Input: dimensioned drawing with shaded views. Units: mm. Origin: part minimum x, y, z. Give positions to 0.01 mm unless a question says otherwise; leave off trailing zeros. Write each loop counter-clockwise with the first axis right and the second up, starting at its lowest first coordinate (ties: lowest second). Pieces come first, ordered by that corner, then holes.
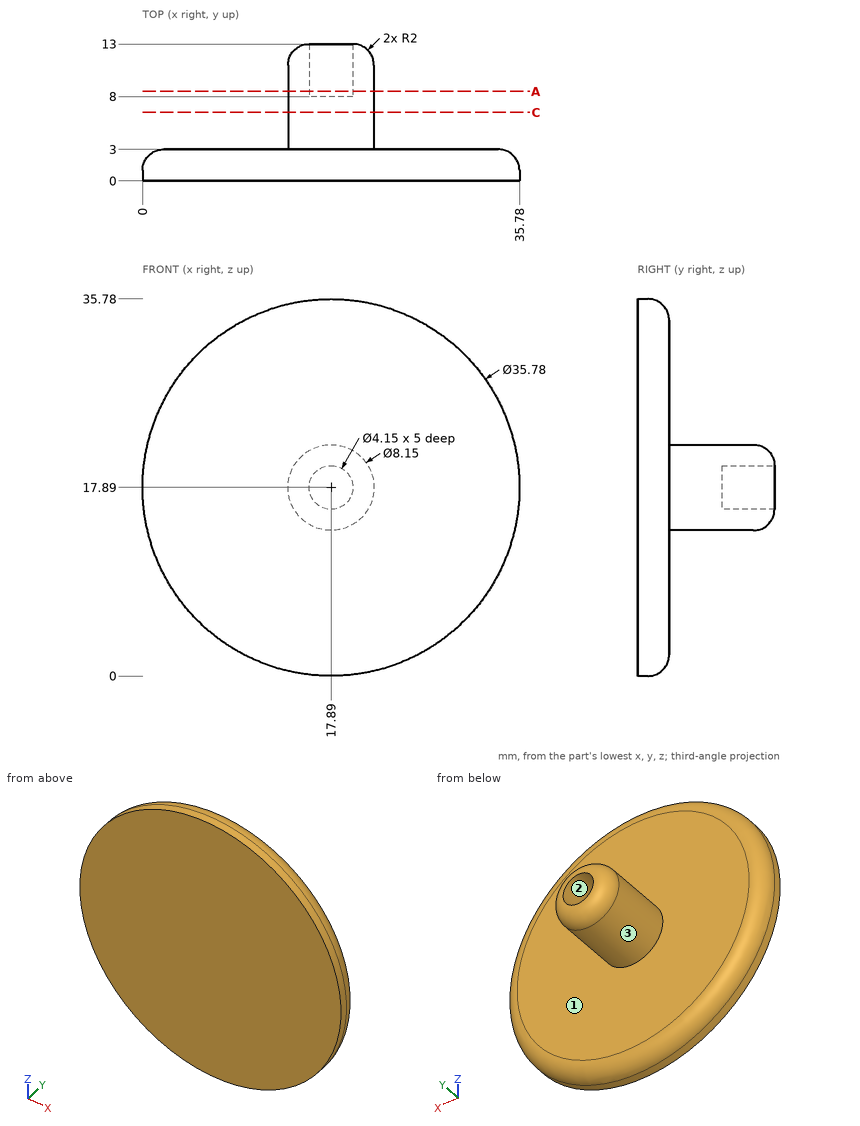
Item 1: Pin query (flat end, axial travel): pin 1 Ø5 at (x, y) = (5.5, 7.5) entering from -Z; pin 2 Ø1.5 at (x, z) = (25.5, 3.5) entering from +Y. Return the tip coordinate at first contact, or that it passes through.
Found:
pin 1: passes through
pin 2: stops at y = 3
Item 2: Section C-C, the plane y = 6.5. Return the cut outline in (x, z) (3 decimals).
Found:
outline: circle Ø8.15 at (17.89, 17.89)
Item 3: Line query: L1, parallel to X at y = 10.9, z = 17.89 (3 decimals); L2, parallel to Z at x = 18, y = 10; L3, parallel to Z at x = 18, y = 3.5. Output: solid intervals per line, ascending.
Found:
L1: x = 13.815 to 15.815, 19.965 to 21.965
L2: z = 13.82 to 15.82, 19.96 to 21.96
L3: z = 13.82 to 21.96
Item 4: Section A-A, the plane y = 8.5. Return the cut outline in (x, z) (3 decimals).
Found:
outline: circle Ø8.15 at (17.89, 17.89); hole circle Ø4.15 at (17.89, 17.89)
Item 5: Pull-direction query (Z, two-part tool) for the marked faces 1, 2 and 3; classes: +Z half, -Z half, draft (parallel to the pull), parting line (faces both ways), or undercut.
Found:
face 1: draft
face 2: undercut
face 3: parting line
